Autodesk Inventor part; units mm, degrees
ref_plane "YZ Plane" through (0, 0, 0) normal (1, 0, 0) x (0, 1, 0)
ref_plane "XZ Plane" through (0, 0, 0) normal (0, 1, 0) x (-1, 0, 0)
ref_plane "XY Plane" through (0, 0, 0) normal (0, 0, 1) x (1, 0, 0)
sketch "Sketch1" plane through (0, 0, 0) normal (0, 0, 1) x (1, 0, 0)
  circle A0 centre (25.4426, 130.4898) radius 3.175
  circle A1 centre (57.1926, 130.4898) radius 3.175
  line L0 (55.6051, 149.5398) -> (27.0301, 149.5398)
  line L1 (41.3176, 149.5398) -> (41.3176, 49.5146)
  arc A2 (61.9551, 49.5146) -> (20.6801, 49.5146) centre (41.3176, 49.5146) ccw
  line L2 (66.7176, 87.6146) -> (66.7176, 149.5398)
  line L3 (15.9176, 87.6146) -> (15.9176, 149.5398)
  line L4 (79.4176, 49.5146) -> (79.4176, 72.4098)
  line L5 (3.2176, 49.5146) -> (3.2176, 72.4098)
  line L6 (66.7176, 149.5398) -> (15.9176, 149.5398)
  line L7 (3.2176, 49.5146) -> (79.4176, 49.5146)
  line L8 (79.4176, 49.5146) -> (79.4176, 74.9146)
  line L9 (3.2176, 49.5146) -> (3.2176, 74.9146)
  arc A3 (15.9176, 87.6146) -> (3.2176, 74.9146) centre (41.3176, 49.5146) ccw
  arc A4 (79.4176, 74.9146) -> (66.7176, 87.6146) centre (41.3176, 49.5146) ccw
  point P0 (27.0301, 149.5398)
  dimension "d2" = 6.35
  dimension "d3" = 6.35
  dimension "d6" = 100.0252
  dimension "d7" = 41.275
  dimension "d18" = 19.05
  dimension "d19" = 19.05
  dimension "d20" = 25.4
  dimension "d21" = 25.4
extrude "Extrusion3" add sketch "Sketch1" along normal blind 12.7 contours L6 L2 A4 L8 L4 L7 A2 L1 L0 | L1 A2 L7 L5 L9 A3 L3 L6 L0
sketch "Sketch2" plane through (79.4176, 49.5146, 0) normal (1, 0, 0) x (0, 0, -1)
  line L0 (0, 0) -> (-12.7, 0)
  line L1 (-6.35, 0) -> (-6.35, 14.3002)
  circle A0 centre (-6.35, 14.3002) radius 3.175
  point P0 (0, -49.5146)
  dimension "d24" = 14.3002
  dimension "d25" = 6.35
extrude "Extrusion4" cut sketch "Sketch2" against normal blind 125.4125
properties part number "Frame Middle"
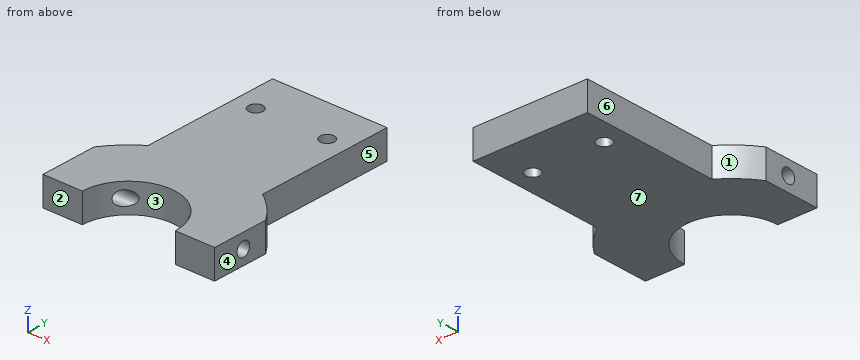
Input: part model. Units: mm. Frame: model coordinates. Face numbers are marked on the shaded views. A direction names the side the tool comes from. Coordinates: 2 decimals unless noted, no trailing zeros. Order: outer loops, then holes, each group sorted by start corner. A loop starts at its lowest first (then second) coordinate and runs counter-clockwise, first axis right, second up. Notation, with made-up numbers: (86.5, -19) - (100.5, -19) arc R4 cw to (100.5, -15) - close; hole circle Ø2 at (61.25, 1). An arc over 180 degrees is marked (long way). Return JSON: item names as keys, results as strings.
Q1. Cut plane D-D (y = 58). Return loops of the section in (x, z).
The answers:
{"outline": "(3.22, 0) - (22.51, 0) - (22.51, 12.7) - (3.22, 12.7) - close; (60.13, 0) - (79.42, 0) - (79.42, 12.7) - (60.13, 12.7) - close"}
Q2. Cut plane B-B (y = 132). Return loops of the section in (x, z).
The answers:
{"outline": "(15.92, 0) - (22.65, 0) - (22.65, 12.7) - (15.92, 12.7) - close; (28.24, 0) - (54.4, 0) - (54.4, 12.7) - (28.24, 12.7) - close; (59.99, 0) - (66.72, 0) - (66.72, 12.7) - (59.99, 12.7) - close"}
Q3. Draft query along X for the marked faces 1, 2, 3 and 4. Return one class per face: +X half, -X half, draft (parallel to the pull), parting line (faces both ways), or undercut.
The answers:
{"face 1": "-X half", "face 2": "draft", "face 3": "undercut", "face 4": "+X half"}
Q4. Access query for the marked faces 5, 6 and 7. Directions: +Z, -Z, +X, -X, +Y, -Y. A direction counts if a zero-diameter tool reaches every point of the face in a straight line with its end or side. Return the directions, or none.
The answers:
{"face 5": "+Z, -Z, +X, +Y", "face 6": "+Z, -Z, -X, +Y", "face 7": "-Z, +X, -X, +Y, -Y"}
Q5. Ray query, probe 1 along Y at (x, z) = (17.5, 6.35); probe 2 along X at (y, z) = (67, 5); probe 3 along X at (y, z) = (105, 1.25). Return the intervals inside material, ascending.
The answers:
{"probe 1": "y = 49.51 to 60.64, 66.99 to 149.54", "probe 2": "x = 3.22 to 30.36, 52.28 to 79.42", "probe 3": "x = 15.92 to 66.72"}
Q6. First-contact query: pin 1 (4 mm diameter, centred on y = 127.5, z = 6.5, fed in from -X); pin 2 (1 mm diameter, centred on y = 98, z = 11, fed in from +X). Flat tips, straight axial feed; report the tip coordinate or a pass-through.
The answers:
{"pin 1": "stops at x = 15.92", "pin 2": "stops at x = 66.72"}
Q7. Cut plane C-C (x = 58). Return loops of the section in (y, z) (3 decimals).
The answers:
{"outline": "(61.664, 0) - (127.419, 0) - (127.419, 12.7) - (61.664, 12.7) - (61.664, 8.685) arc R3.175 cw (long way) to (61.664, 4.015) - close; (133.56, 0) - (149.54, 0) - (149.54, 12.7) - (133.56, 12.7) - close"}
Q8. Cut plane A-A (z = 6.35). State how many separate pieces and enclosed holes the cut face has, then the cut area to 3 significant figures.
The answers:
{"separate pieces": "3", "enclosed holes": "2", "area": "4,880 mm2"}
